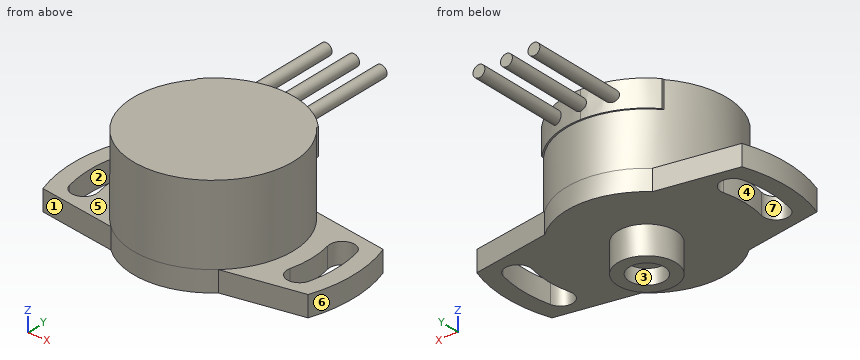
```python
from build123d import *
from build123d.topology import SkipClean

# Parameters (mm, degrees)
SKETCH1_R           = 13.716
BOSS_EXTRUDE1_DEPTH = 13.589
BOSS_EXTRUDE2_START = 3.556
BOSS_EXTRUDE2_DEPTH = 3.556
CUT_EXTRUDE1_DEPTH  = 3.556
SKETCH4_R           = 4.953
BOSS_EXTRUDE3_DEPTH = 4.826
SKETCH5_R           = 3.01625
CUT_EXTRUDE2_DEPTH  = 2.54
BOSS_EXTRUDE4_START = -4.572
BOSS_EXTRUDE4_DEPTH = 4.572
SKETCH6_R           = 1.016
BOSS_EXTRUDE5_DEPTH = 29.464


with BuildPart() as part:
    # Sketch1 → Boss-Extrude1 (new body)
    with BuildSketch(Plane.XY):
        Circle(SKETCH1_R)
    extrude(amount=BOSS_EXTRUDE1_DEPTH)

    # Sketch2 → Boss-Extrude2 (add)
    with BuildSketch(Plane(origin=(0, 0, 0), x_dir=(-1, 0, 0), z_dir=(0, 0, -1)).offset(BOSS_EXTRUDE2_START)):
        with BuildLine():
            Line((-9.214285431, 10.16), (-22.674746592, 7.874))
            ThreePointArc((-22.674746592, 7.874), (-24.003, 0), (-22.674746592, -7.874))
            Line((-22.674746592, -7.874), (-9.214285431, -10.16))
            ThreePointArc((-9.214285431, -10.16), (13.716, 0), (-9.214285431, 10.16))
        make_face()
    boss_extrude2 = extrude(amount=-BOSS_EXTRUDE2_DEPTH)

    # Sketch3 → Cut-Extrude1 (cut)
    with BuildSketch(Plane(origin=(0, 0, -3.556), x_dir=(-1, 0, 0), z_dir=(0, 0, -1))):
        with BuildLine():
            ThreePointArc((-16.365965281, -3.96831406), (-16.8402, 6.1e-08), (-16.365965252, 3.968314178))
            ThreePointArc((-16.365965252, 3.968314178), (-17.93670842, 6.544602887), (-20.512997182, 4.973859806))
            ThreePointArc((-20.512997182, 4.973859806), (-21.1074, 4.2e-08), (-20.512997202, -4.973859724))
            ThreePointArc((-20.512997202, -4.973859724), (-17.936708402, -6.544602882), (-16.365965281, -3.96831406))
        make_face()
    cut_extrude1 = extrude(amount=-CUT_EXTRUDE1_DEPTH, mode=Mode.SUBTRACT)

    # Mirror1: Boss-Extrude2, Cut-Extrude1 across plane
    add(boss_extrude2.mirror(Plane(origin=(0, 0, 0), x_dir=(0, 0, 1), z_dir=(1, 0, 0))))
    add(cut_extrude1.mirror(Plane(origin=(0, 0, 0), x_dir=(0, 0, 1), z_dir=(1, 0, 0))), mode=Mode.SUBTRACT)

    # Sketch4 → Boss-Extrude3 (add)
    with BuildSketch(Plane(origin=(0, 0, -3.556), x_dir=(-1, 0, 0), z_dir=(0, 0, -1))):
        Circle(SKETCH4_R)
    extrude(amount=BOSS_EXTRUDE3_DEPTH)

    # Sketch5 → Cut-Extrude2 (cut)
    with BuildSketch(Plane(origin=(0, 0, -8.382), x_dir=(-1, 0, 0), z_dir=(0, 0, -1))):
        Circle(SKETCH5_R)
    extrude(amount=-CUT_EXTRUDE2_DEPTH, mode=Mode.SUBTRACT)

    # Sketch7 → Boss-Extrude4 (add)
    with BuildSketch(Plane.XY.offset(13.589).offset(BOSS_EXTRUDE4_START)):
        with BuildLine():
            Line((0, 5.951559827), (0, 13.716))
            ThreePointArc((0, 13.716), (-5.643281246, 12.501281246), (-10.287, 9.072281246))
            Line((-10.287, 9.072281246), (-10.287, 5.951559827))
            Line((-10.287, 5.951559827), (0, 5.951559827))
        make_face()
        with BuildLine():
            Line((10.287, 5.951559827), (10.287, 9.072281246))
            ThreePointArc((10.287, 9.072281246), (5.643281246, 12.501281246), (0, 13.716))
            Line((0, 13.716), (0, 5.951559827))
            Line((0, 5.951559827), (10.287, 5.951559827))
        make_face()
        with BuildLine():
            Line((0, 13.716), (0, 13.97))
            ThreePointArc((0, 13.97), (-5.617729535, 12.790700328), (-10.287, 9.45190621))
            Line((-10.287, 9.45190621), (-10.287, 9.072281246))
            ThreePointArc((-10.287, 9.072281246), (-5.643281246, 12.501281246), (0, 13.716))
        make_face()
        with BuildLine():
            Line((10.287, 9.072281246), (10.287, 9.45190621))
            ThreePointArc((10.287, 9.45190621), (5.617729535, 12.790700328), (0, 13.97))
            Line((0, 13.97), (0, 13.716))
            ThreePointArc((0, 13.716), (5.643281246, 12.501281246), (10.287, 9.072281246))
        make_face()
    extrude(amount=BOSS_EXTRUDE4_DEPTH)

    # Sketch6 → Boss-Extrude5 (add)
    with SkipClean():  # the faces are left unmerged after this step: merging them gives an invalid solid
        with BuildSketch(Plane(origin=(0, 0, 0), x_dir=(1, 0, 0), z_dir=(0, 1, 0))):
            with Locations(Location((0, -11.303, 0), (0, 0, 90))):
                Circle(SKETCH6_R)
            with Locations(Location((-4.699, -11.303, 0), (0, 0, 90))):
                Circle(SKETCH6_R)
            with Locations(Location((4.699, -11.303, 0), (0, 0, 90))):
                Circle(SKETCH6_R)
        extrude(amount=BOSS_EXTRUDE5_DEPTH)


solid = part.part
```
Input: part model. Units: mm. Frame: model coordinates. Face numbers are marked on the shaded views. A direction names the side the tool comes from. Give positions to 0.01 mm unless a question says otherwise; leave off trailing zeros. Order: outer loops, then holes, each group sorted by start corner. A loop starts at its lowest first (then second) coordinate and runs counter-clockwise, first axis right, second up. Notation, with made-up numbers: M -33.5,89 L 0.5,89 A16 cw 0.5,116 Z; hole C 76,31 d2. An arc over 180 degrees is marked long. Return JSON: item names as keys, results as strings.
1) Access query for the marked faces 1, 2 and 3. Directions: +Z, -Z, +X, -X, +Y, -Y. A direction counts if a zero-diameter tool reaches every point of the face in a straight line with its end or side. Return the directions, or none.
Taken from the geometry:
{"face 1": "+Z, -Z, -X, -Y", "face 2": "+Z, -Z", "face 3": "-Z"}
2) Mould query, pull axis Y, two halves, no side actions, for the marked faces 4, 5, 6 and 7. Classes: released by +Y, released by -Y, zero draft, split by the parting line, or undercut.
Taken from the geometry:
{"face 4": "undercut", "face 5": "zero draft", "face 6": "split by the parting line", "face 7": "undercut"}
3) Section query B-B on x = -19.5. Output: boundary loops of the cut face in (y, z), and give its area (3 significant figures).
Taken from the geometry:
{"outline": "M -8.41,-3.56 L -6.32,-3.56 L -6.32,0 L -8.41,0 Z; M 6.32,-3.56 L 8.41,-3.56 L 8.41,0 L 6.32,0 Z", "area": "14.9 mm2"}
4) Section query A-A on y = 0. Output: boundary loops of the cut face in (x, z).
Taken from the geometry:
{"outline": "M -24,-3.56 L -21.11,-3.56 L -21.11,0 L -24,0 Z; M -16.84,-3.56 L -4.95,-3.56 L -4.95,-8.38 L -3.02,-8.38 L -3.02,-5.84 L 3.02,-5.84 L 3.02,-8.38 L 4.95,-8.38 L 4.95,-3.56 L 16.84,-3.56 L 16.84,0 L 13.72,0 L 13.72,13.59 L -13.72,13.59 L -13.72,0 L -16.84,0 Z; M 21.11,-3.56 L 24,-3.56 L 24,0 L 21.11,0 Z"}
5) Section query D-D on y = 11.5. Output: boundary loops of the cut face in (x, z), and give its area (3 significant figures).
Taken from the geometry:
{"outline": "M -7.93,9.02 L -7.48,9.02 L -7.48,-3.56 L 7.48,-3.56 L 7.48,9.02 L 7.93,9.02 L 7.93,13.59 L -7.93,13.59 Z", "area": "260 mm2"}
6) Contact query for flat-ended pins moving along their axis: pin 1 (4 mm diameter, centred on y = -5, z = 3, fed in from +X); pin 2 (10 mm diameter, centred on x = 11, z = 8, fed in from -Y); pin 3 (5.5 mm diameter, centred on x = 4.5, y = 10.5, fed in from -Z). Output: stop coordinate, or through.
Taken from the geometry:
{"pin 1": "stops at x = 13.38", "pin 2": "stops at y = -12.33", "pin 3": "stops at z = -3.56"}
7) Line query: L1, parallel to Y at x = 0, z = -7.8; L2, parallel to Z at x = 21.5, y = -5.5; L3, parallel to Z at x = -3, y = -4.5. Output: solid intervals per line, ascending. Write a range as [from, to].
Taken from the geometry:
{"L1": "y = [-4.95, -3.02], [3.02, 4.95]", "L2": "z = [-3.56, 0]", "L3": "z = [-3.56, 13.59]"}
8) Section query C-C on z = 3. Output: boundary loops of the cut face in (x, y), and give its area (3 significant figures).
Taken from the geometry:
{"outline": "C 0,0 d27.43", "area": "591 mm2"}
